Can you work these out from the model? Positions are in its coordinate system, mm. Face numbers are marked on the shaded views. A direction names the side the tool comes from. Coordinates: 2 decimals unless noted, no trailing zeros. Order: outer loops, then holes, each group sorted by start corner. A loop starts at its lowest first (then second) coordinate and runs counter-clockwise, first axis right, second up. Notation, with made-up numbers: (31, 5) -> (40, 5) arc R34 cw to (40, 43) -> close; hole circle Ø7 at (70, 60). An arc over 180 degrees is marked (long way). Write item = value, one per line. Start each with the question number.
from build123d import *

# Parameters (mm, degrees)
SKETCH1_R           = 3
BOSS_EXTRUDE1_DEPTH = 7
CHAMFER1_SIZE       = 1
CHAMFER1_SIZE2      = 0.363970234
SKETCH2_R           = 3.25
BOSS_EXTRUDE3_DEPTH = 1
SKETCH4_R           = 3
BOSS_EXTRUDE4_DEPTH = 5.2
CHAMFER2_SIZE       = 2.25
CHAMFER2_SIZE2      = 0.818933027
SKETCH2_2_R         = 3.25
BOSS_EXTRUDE5_DEPTH = 1


with BuildPart() as part:
    # Sketch1 → Boss-Extrude1 (new body)
    with BuildSketch(Plane.XY):
        Circle(SKETCH1_R)
    extrude(amount=BOSS_EXTRUDE1_DEPTH)

    # Chamfer1
    chamfer1_edges = [part.edges().sort_by_distance(p)[0] for p in [
        (-3, 0, 7),
    ]]
    chamfer1_side = [part.faces().sort_by_distance(p)[0] for p in [
        (-3, 0, 3.5),
    ]]
    chamfer(chamfer1_edges, length=CHAMFER1_SIZE, length2=CHAMFER1_SIZE2, reference=chamfer1_side[0])

    # Sketch2 → Boss-Extrude3 (add)
    with BuildSketch(Plane(origin=(0, 0, 0), x_dir=(-1, 0, 0), z_dir=(0, 0, -1))):
        Circle(SKETCH2_R)
    extrude(amount=BOSS_EXTRUDE3_DEPTH)

    # Sketch4 → Boss-Extrude4 (add)
    with BuildSketch(Plane(origin=(0, 0, -1), x_dir=(-1, 0, 0), z_dir=(0, 0, -1))):
        Circle(SKETCH4_R)
    extrude(amount=BOSS_EXTRUDE4_DEPTH)

    # Chamfer2
    chamfer2_edges = [part.edges().sort_by_distance(p)[0] for p in [
        (3, 0, -6.2),
    ]]
    chamfer2_side = [part.faces().sort_by_distance(p)[0] for p in [
        (3, 0, -3.6),
    ]]
    chamfer(chamfer2_edges, length=CHAMFER2_SIZE, length2=CHAMFER2_SIZE2, reference=chamfer2_side[0])

    # Sketch2_2 → Boss-Extrude5 (add)
    with BuildSketch(Plane(origin=(0, 0, 0), x_dir=(-1, 0, 0), z_dir=(0, 0, -1))):
        Circle(SKETCH2_2_R)
    extrude(amount=BOSS_EXTRUDE5_DEPTH)


solid = part.part
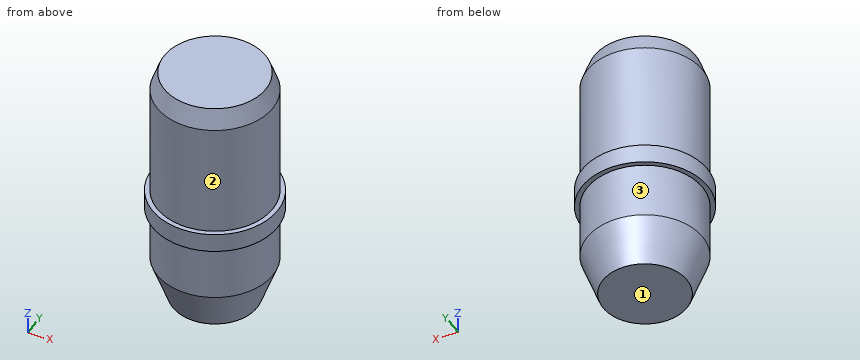
(1) For the marked faces 1, 2 and 3, which set-ups out of +Z, -Z, +X, -X, +Y, -Y let a thin tool reach every point of the face, with its end or its side?
(2) Imagine slicing it at A-A (x = 0). Write out the boundary of the cut face in (y, z), plus the area to 3 significant figures.
(3) For P1, Ø3, axis at x = 2, z = 5, coming from the -Y side; P2, Ø1, axis at y = -0.5, z = 2.5, coming from the +X side, each with a flat end and sliding along its axis, tell me the tip position at first contact or that it passes through.
(4) If I drill on L1, parallel to Z at x = -1.5, y = 2.75; L2, parallel to Y at x = -1.5, z = 3.5; L3, parallel to Y at x = -0.75, z = 1, over which ranges is the centre line in solid material (lowest first)? Write a range as from..to.
(5) Imagine slicing it at D-D (z = -5.5). Write out the boundary of the cut face in (x, y).
(6) Imagine slicing it at C-C (z = -1.5). Write out the boundary of the cut face in (x, y).
Result set:
q1.face_1 = -Z, +X, -X, +Y, -Y
q1.face_2 = +Z
q1.face_3 = -Z
q2.outline = (-3.25, -1) -> (-3, -1) -> (-3, -3.95) -> (-2.18, -6.2) -> (2.18, -6.2) -> (3, -3.95) -> (3, -1) -> (3.25, -1) -> (3.25, 0) -> (3, 0) -> (3, 6) -> (2.64, 7) -> (-2.64, 7) -> (-3, 6) -> (-3, 0) -> (-3.25, 0) -> close
q2.area = 77.5 mm2
q3.P1 = -2.96
q3.P2 = 3
q4.L1 = -1..0
q4.L2 = -2.6..2.6
q4.L3 = -2.9..2.9
q5.outline = circle Ø4.87 at (0, 0)
q6.outline = circle Ø6 at (0, 0)
